```python
from build123d import *

# Parameters (mm, degrees)
SKETCH1_R            = 127
BOSS_EXTRUDE1_DEPTH  = 3.175
M3_CLEARANCE_HOLE1_D = 3.4
CIRPATTERN1_COUNT    = 8
BOSS_EXTRUDE2_DEPTH  = 3.175
CIRPATTERN2_COUNT    = 8


with BuildPart() as part:
    # Sketch1 → Boss-Extrude1 (new body)
    with BuildSketch(Plane.XY):
        Circle(SKETCH1_R)
    extrude(amount=BOSS_EXTRUDE1_DEPTH)

    # M3 Clearance Hole1 (through all)
    with Locations(Plane(origin=(0, 0, 0), x_dir=(-1, 0, 0), z_dir=(0, 0, -1))):
        with Locations((-58.2494214, 58.493652703), (-82.549819355, -0.172697611), (-93.238867767, 66.113565457), (-112.679186132, 19.180485205), (-11.733270063, 4.860079591), (-68.767621753, 45.667457762), (-80.917820731, 16.334282605), (-35.199810189, 14.580238773)):
            m3_clearance_hole1 = Hole(M3_CLEARANCE_HOLE1_D / 2)

    # CirPattern1: M3 Clearance Hole1 ×8 about axis
    cirpattern1_axis = Axis((-0.09749486, -0.040383693, 0), (0, 0, 1))
    for i in range(1, CIRPATTERN1_COUNT):
        add(m3_clearance_hole1.rotate(cirpattern1_axis, i * 360 / CIRPATTERN1_COUNT), mode=Mode.SUBTRACT)

    # Sketch6 → Boss-Extrude2 (add)
    with BuildSketch(Plane(origin=(0, 0, 0), x_dir=(-1, 0, 0), z_dir=(0, 0, -1))):
        with BuildLine():
            Line((-100.530886518, 72.570613756), (-138.664014222, 88.365872427))
            ThreePointArc((-138.664014222, 88.365872427), (-160.534372382, 88.365872427), (-175.999050943, 72.901193866))
            Line((-175.999050943, 72.901193866), (-186.934230023, 46.501336224))
            Line((-186.934230023, 46.501336224), (-122.401244677, 19.770898473))
            Line((-122.401244677, 19.770898473), (-100.530886518, 72.570613756))
        make_face()
    boss_extrude2 = extrude(amount=-BOSS_EXTRUDE2_DEPTH)

    # CirPattern2: Boss-Extrude2 ×8 about axis
    cirpattern2_axis = Axis((0, 0, 0), (0, 0, 1))
    for i in range(1, CIRPATTERN2_COUNT):
        add(boss_extrude2.rotate(cirpattern2_axis, i * 360 / CIRPATTERN2_COUNT))


solid = part.part
```
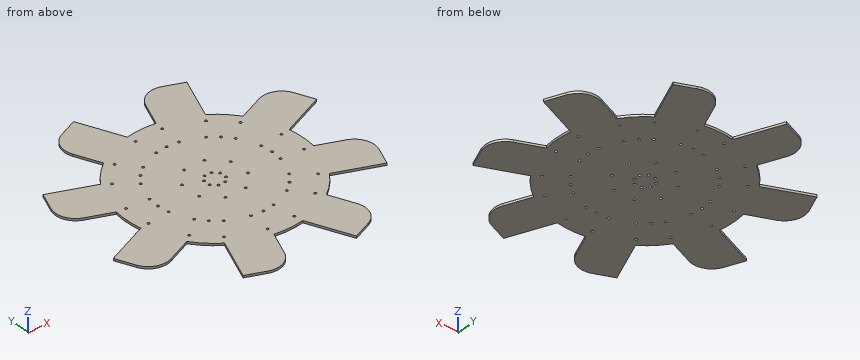
Verification items for the finished model (mm, model axes). Round coordinates to 2 decimals unless told otherwise and drop trailing zeros. Order: outer loops, then holes, each group sorted by start corner. A loop starts at its lowest first (then second) coordinate and runs counter-clockwise, first axis right, second up.
1) Cross-section at B-B, the plane z = 2.1. Give the number of separate pieces and of enclosed holes in the cut face, plus the area to 3 significant figures.
Geometry says:
separate pieces: 1
enclosed holes: 56
area: 78,300 mm2
2) Material ranges on line 1 (Y direction, x = -17, z = 1.9); line 2 (X direction, y = 66, z = 1.1); line 3 (Y direction, x = -59, z = 1.9), recorded low to high.
Geometry says:
line 1: y = -125.86 to -82.67, -79.44 to 79.36, 82.59 to 125.86
line 2: x = -177.89 to -95.13, -91.74 to 91.54, 94.94 to 178.86
line 3: y = -178.02 to -60.18, -56.73 to 56.65, 60.1 to 181.76
3) Depth check by flat-ended pin: pin 1 (1.5 mm diameter, centred on y = 43.5, z = 1.5, fed in from +X); pin 2 (1 mm diameter, centred on y = 91, z = 2, fed in from -X). Enter the tip coordinate at first touch or a pass-through.
Geometry says:
pin 1: stops at x = 181.5
pin 2: stops at x = -168.71
4) Cross-section at A-A, the plane y = -154.5. Record the cut outline in (x, z) (3 decimals).
Geometry says:
outline: (-94.925, 0) - (-33.067, 0) - (-33.067, 3.175) - (-94.925, 3.175) - close; (33.067, 0) - (90.118, 0) - (90.118, 3.175) - (33.067, 3.175) - close
